Part model, mm, in its own coordinate system. A direction names the side the tool comes from. Coordinates: 2 decimals unless noted, no trailing zeros. Loops run counter-clockwise (first coordinate to the right, second up) from the corner with the lowest first, then second, coordinate; pieces in that order, holes last. Notation, with made-up numbers: M 70.25,-10 L 108.25,-10 A16 ccw 108.25,18 Z; hole C -14.5,-11.5 d11. An arc over 180 degrees is marked long. Answer as a JSON object with one key per item and string values. Group by question number.
1. Drop flat-ended pins along their axis: pin 1 Ø7.5 at (y, z) = (23, 68) entering from -X; pin 2 Ø10 at (x, z) = (27, 65) entering from -Y; pin 3 Ø1.5 at (x, y) = (45, 29) entering from -Z; pin 4 Ø5.5 at (y, z) = (43.053, 111.125) entering from +X. Give the stop position or say it passes through.
2. Saw through at D-D on z = 84. Write the cut outline in (x, y).
3. Saw through at B-B on y = 18.5. Write the cut outline in (x, z) (3 decimals), then the cut area to 3 significant figures.
4. Saw through at A-A on x = 14. Write the cut outline in (y, z) (3 decimals), then the cut area to 3 significant figures.
5. 3-axis set-ups, long thin cutter, end or side, ignore diameter. For faces 1 (the face through (43.56, 27.69, 7.64)), 2 (the face through (34.798, 28, 66)), 3 (the face through (8.94, 41.45, 21)): which of +Z, -Z, +X, -X, +Y, -Y reach the whole face in a straight line?
6. Saw through at C-C on x = 31. Write the cut outline in (y, z), then the cut area to 3 significant figures.
7. Drill centre lines: L1, parallel to Z at x = 16.5, y = 32 (3 decimals); L2, parallel to X at y = 45, z = 72; L3, parallel to Y at x = 8, z = 23.5. Where is each one in solid material? Low to high.
8. Mould opens along Y. For faces 4 (the face through (36, 0, 66)), 5 (the face through (8.937, 41.565, 112.49)), 6 (the face through (13, 28, 0)) say: released by +Y, released by -Y, zero draft, split by the parting line, or undercut.
from build123d import *

# Parameters (mm, degrees)
F0_W     = 50.8
F0_H     = 54.61
F1_DEPTH = 133.35
F3_D     = 4.0386
F3_DEPTH = 17.6276
F3_TIP   = 1.213317848
F5_DEPTH = 54.611


with BuildPart() as f1:
    # F0 (on Top) → F1 (new body)
    with BuildSketch(Plane.XY):
        with Locations((25.4, 27.305)):
            Rectangle(F0_W, F0_H)
    extrude(amount=F1_DEPTH)

    # F3
    with Locations(Plane(origin=(0, 0, 0), x_dir=(0, -1, 0), z_dir=(-1, 0, 0))):
        with Locations((-11.557, 22.225), (-43.053, 22.225), (-11.557, 111.125), (-43.053, 111.125)):
            Hole(F3_D / 2, depth=F3_DEPTH)
            with Locations((0, 0, -(F3_DEPTH + F3_TIP / 2))):  # 118° drill point
                Cone(0, F3_D / 2, F3_TIP, mode=Mode.SUBTRACT)

    # F4 (on face) → F5 (intersect, through all)
    with BuildSketch(Plane(origin=(0, 54.61, 0), x_dir=(-1, 0, 0), z_dir=(0, 1, 0))):
        with BuildLine():
            Line((-22.098, 92.075), (0, 92.075))
            Line((0, 92.075), (0, 133.35))
            Line((0, 133.35), (-25.4, 133.35))
            ThreePointArc((-25.4, 133.35), (-43.3605122421, 125.9105122421), (-50.8, 107.95))
            Line((-50.8, 107.95), (-50.8, 25.4))
            ThreePointArc((-50.8, 25.4), (-43.3605122421, 7.4394877579), (-25.4, 0))
            Line((-25.4, 0), (0, 0))
            Line((0, 0), (0, 41.275))
            Line((0, 41.275), (-22.098, 41.275))
            ThreePointArc((-22.098, 41.275), (-31.0782561211, 44.9947438789), (-34.798, 53.975))
            Line((-34.798, 53.975), (-34.798, 79.375))
            ThreePointArc((-34.798, 79.375), (-31.0782561211, 88.3552561211), (-22.098, 92.075))
        make_face()
    extrude(amount=-F5_DEPTH, mode=Mode.INTERSECT)


solid = f1.part
Outcome:
{
 "1": {"pin 1": "stops at x = 34.8", "pin 2": "passes through", "pin 3": "stops at z = 8.38", "pin 4": "stops at x = 50.8"},
 "2": {"outline": "M 33.93,0 L 50.8,0 L 50.8,54.61 L 33.93,54.61 Z"},
 "3": {"outline": "M 0,0 L 25.4,0 A25.4 ccw 50.8,25.4 L 50.8,107.95 A25.4 ccw 25.4,133.35 L 0,133.35 L 0,92.075 L 22.098,92.075 A12.7 cw 34.798,79.375 L 34.798,53.975 A12.7 cw 22.098,41.275 L 0,41.275 Z", "area": "4,800 mm²"},
 "4": {"outline": "M 0,0 L 54.61,0 L 54.61,41.275 L 0,41.275 Z; M 0,92.075 L 54.61,92.075 L 54.61,133.35 L 0,133.35 Z; hole C 11.557,22.225 d4.039; hole C 11.557,111.125 d4.039; hole C 43.053,22.225 d4.039; hole C 43.053,111.125 d4.039", "area": "4,460 mm²"},
 "5": {"face 1": "-Z, +X, +Y, -Y", "face 2": "-X, +Y, -Y", "face 3": "-X"},
 "6": {"outline": "M 0,0.63 L 54.61,0.63 L 54.61,44.92 L 0,44.92 Z; M 0,88.43 L 54.61,88.43 L 54.61,132.72 L 0,132.72 Z", "area": "4,840 mm²"},
 "7": {"L1": "z = 0 to 41.275, 92.075 to 133.35", "L2": "x = 34.8 to 50.8", "L3": "y = 0 to 9.99, 13.12 to 41.49, 44.62 to 54.61"},
 "8": {"face 4": "released by -Y", "face 5": "undercut", "face 6": "zero draft"}
}
